from build123d import *

# Parameters (mm, degrees)
ZAOBLIT1_R   = 0.294
ZKOSIT1_SIZE = 0.147
ZAOBLIT2_R   = 0.3528


with BuildPart() as part:
    # Skica1 → Otočit kolem osy1 (revolve)
    with BuildSketch(Plane.XY, mode=Mode.PRIVATE) as oto_it_kolem_osy1_sk:
        Polygon((0, 5), (3.5, 5), (3.5, 3.327141994), (4.2, 3.07236283), (4.2, 2.5), (3.375703588, 2.92), (1.26, 2.92), (0.42, 2.5), (0.168, 2.752), (0.168, 3.222223069), (2.333333333, 3.802422387), (0, 4.42763717), align=None)
    revolve(oto_it_kolem_osy1_sk.sketch.rotate(Axis((0, 0, 0), (1, 0, 0)), 90), axis=Axis((0, 0, 0), (1, 0, 0)))

    # Zaoblit1
    zaoblit1_edges = [part.edges().sort_by_distance(p)[0] for p in [
        (2.333333333, 0, -3.802422387),
    ]]
    fillet(zaoblit1_edges, radius=ZAOBLIT1_R)

    # Zkosit1
    zkosit1_edges = [part.edges().sort_by_distance(p)[0] for p in [
        (3.5, 0, -5),
        (0, 0, -5),
    ]]
    chamfer(zkosit1_edges, length=ZKOSIT1_SIZE)

    # Zaoblit2
    zaoblit2_edges = [part.edges().sort_by_distance(p)[0] for p in [
        (3.5, 0, -3.327141994),
    ]]
    fillet(zaoblit2_edges, radius=ZAOBLIT2_R)


solid = part.part
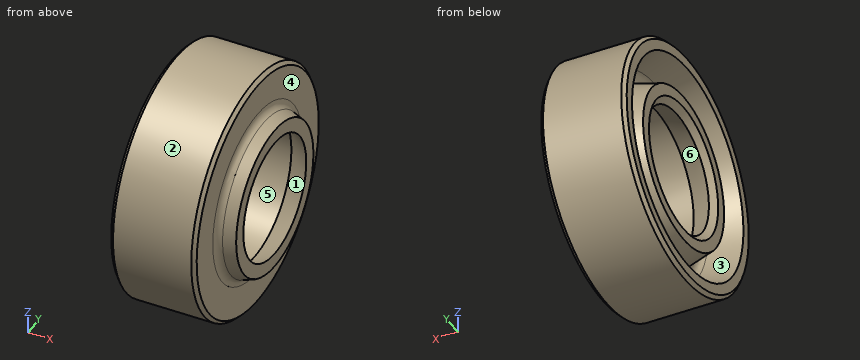
Read the model definition and answer for the solid it produces. Units are mm, in the model's axes. Face numbers are marked on the shaded views. A direction names the side the tool comes from. Coordinates: 2 decimals unless noted, no trailing zeros. Loops run counter-clockwise (first coordinate to the right, second up) from the corner with the lowest first, then second, coordinate; pieces in that order, holes last.
Q1. The part is cut by section A-A on x = 2.25. Write down the section's boundary in (y, z), and give its area (3 significant figures).
Q2. Which of the six approach directions +Z, -Z, +X, -X, +Y, -Y give full straight-line access (tool end or side, diameter ignored) to the marked faces 1 and 2?
Q3. Each of these flat-tipped pins is pushed along its axis until it touches: pin 1 Ø3 at (y, z) = (1, -1) entering from -X; pin 2 Ø2 at (x, z) = (2.5, -2.5) entering from +Y. Where does it stop, or does it pass through?
Q4. Consider probe 1 along Y at (x, z) = (2.65, 0); probe 2 along Z at (x, y) = (0.7, 2.25); probe 3 along Z at (x, y) = (1.2, -1). Determine where each line is inside the solid, lowest interval first.
Q5. The mould has two halves that part along X. Classify the marked faces 3, 4, 5 and 6: +X half, -X half, draft (parallel to the pull), parting line (faces both ways), or undercut.
Q6. The part is cut by section B-B on x = 0.8. Write down the section's boundary in (y, z), and give its area (3 significant figures).
Results below:
1. outline: circle Ø10 at (0, 0); hole circle Ø5.84 at (0, 0)
1. area: 51.8 mm2
2. face 1: none
2. face 2: +X, -X
3. pin 1: stops at x = 0.17
3. pin 2: stops at y = 4.77
4. probe 1: y = -5 to -2.92, 2.92 to 5
4. probe 2: z = -4.47 to -3.59, -2.5 to -1.38, 1.38 to 2.5, 3.59 to 4.47
4. probe 3: z = -4.9 to -3.98, -3.35 to -2.71, 2.71 to 3.35, 3.98 to 4.9
5. face 3: -X half
5. face 4: +X half
5. face 5: undercut
5. face 6: undercut
6. outline: circle Ø10 at (0, 0); circle Ø6.78 at (0, 0); hole circle Ø8.43 at (0, 0); hole circle Ø5.38 at (0, 0)
6. area: 36.2 mm2
